```python
from build123d import *

# Parameters (mm, degrees)
F0_W     = 330
F0_H     = 370
F1_DEPTH = 35.56
F2_W     = 80
F2_H     = 85
F3_DEPTH = 17
F4_R     = 5.431647
F4_R_2   = 7.363502
F4_R_3   = 7.681498
F4_R_4   = 6.500814
F5_DEPTH = 18.561


with BuildPart() as f1:
    # F0 (on Top) → F1 (new body)
    with BuildSketch(Plane.XY):
        with Locations((0, -185)):
            Rectangle(F0_W, F0_H)
    extrude(amount=F1_DEPTH)

    # F2 (on face) → F3 (cut)
    with BuildSketch(Plane.XY.offset(35.56)):
        with Locations((0, -42.5)):
            Rectangle(F2_W, F2_H)
    extrude(amount=-F3_DEPTH, mode=Mode.SUBTRACT)

    # F4 (on face) → F5 (cut, through all)
    with BuildSketch(Plane.XY.offset(18.56)):
        with Locations((-24.62519, -16.512778)):
            Circle(F4_R)
        with Locations((17.679622, -23.458349)):
            Circle(F4_R_2)
        with Locations((-24.62519, -63.237496)):
            Circle(F4_R_3)
        with Locations((15.785381, -62.606081)):
            Circle(F4_R_4)
    extrude(amount=-F5_DEPTH, mode=Mode.SUBTRACT)


solid = f1.part
```
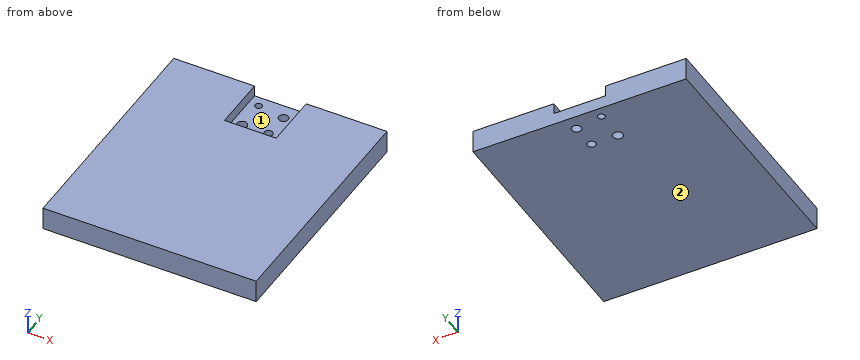
Here's how the part is built. I have some questions about the finished solid (model axes, mm). Face numbers are marked on the shaded views. Give positions to 0.01 mm unless a question says otherwise; leave off trailing zeros. Loops run counter-clockwise (first coordinate to the right, second up) from the corner with the lowest first, then second, coordinate; pieces in that order, holes last. Notation, with made-up numbers: M 30,78.25 L 80,78.25 A18 cw 80,91.25 Z; hole C 62,37.25 d7. An arc over 180 degrees is marked long. Put each result on its own line as item: value. Start each with the question number.
(1) I want a section at A-A on z = 25. Please give me the cut outline in (x, y), then the cut area to 3 significant figures.
(2) Will these pins go through, and if not, where does the flat tip stop? pin 1 Ø12 at (x, y) = (17.68, -23.46) entering from -Z; pin 2 Ø8.5 at (x, z) = (-5.5, 26.5) entering from +Y; pin 3 Ø1 at (x, z) = (-0.5, 15.5) entering from +Y; pin 4 Ø15 at (x, y) = (15.79, -62.61) entering from +Z.
(3) I need wall thicknesses on line 1 along Z through (x, y) = (-20.5, -33). Which ranges of the line are inside material? Lowest first, please. Write a range as [from, to].
(4) If we mould it in two halves opening along X, with no side actions, what happens to the marked faces 1 and 2? For each: +X half, -X half, draft (parallel to the pull), parting line (faces both ways), or undercut.
Answer block:
1. outline: M -165,-370 L 165,-370 L 165,0 L 40,0 L 40,-85 L -40,-85 L -40,0 L -165,0 Z
1. area: 115,000 mm^2
2. pin 1: through
2. pin 2: y = -85
2. pin 3: y = 0
2. pin 4: z = 18.56
3. line 1: [0, 18.56]
4. face 1: undercut
4. face 2: draft
